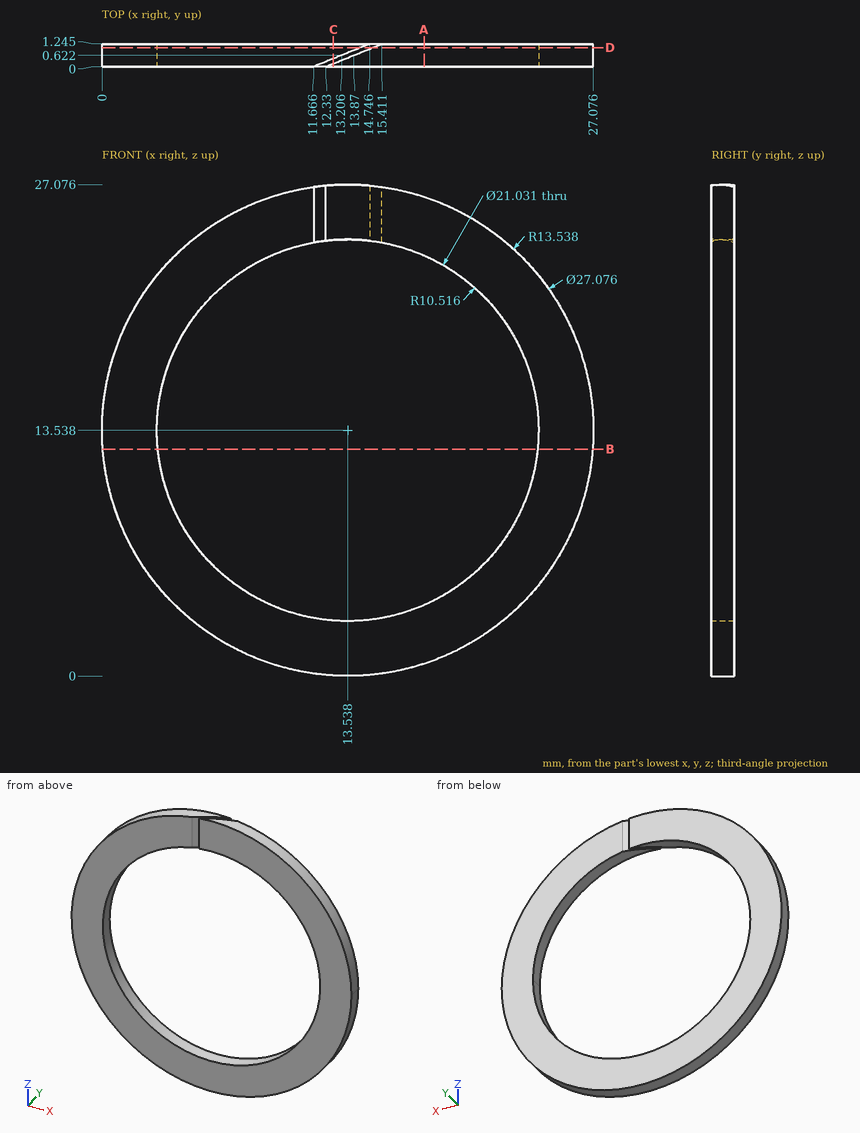
Answer from the drawing. Dimensions are ordinates in mm from the lowest x, y and z of the part. Coordinates: 2 decimals unless noted, no trailing zeros. Loops run counter-clockwise (first coordinate to the right, second up) from the corner with the lowest first, then second, coordinate; pieces in that order, holes last. Notation, with made-up numbers: (63.25, 7.5) -> (85.25, 7.5) arc R16 ccw to (85.25, 34.5) -> close; hole circle Ø1 at (44.25, -17.5). An arc over 180 degrees is marked (long way). Answer in a Markdown table with one row per item.
Item 1: This flat-tipped pin is pushed along its axis until it touches: P1, Ø12, axis at x = 17.5, z = 15.5, coming from the -Y side. Where does it stop, or does it pass through?
Returned:
| item | result |
|---|---|
| P1 | passes through |
Item 2: A cutting plane is placed at B-B on z = 12.5. Determine the outline of the cut face in (x, y) (1 decimal).
Returned:
| item | result |
|---|---|
| outline | (0, 0) -> (3.1, 0) -> (3.1, 1.2) -> (0, 1.2) -> close; (24, 0) -> (27, 0) -> (27, 1.2) -> (24, 1.2) -> close |
Item 3: Straight lines are drawn through the part: line 1 along Z through (x, y) = (13.5, 0.85); line 2 along Z through (x, y) = (17.25, 0.65); line 3 along X through (y, z) = (1, 19.5) (1 decimal). For each, find the intervals that lie inside material, in ascending order. Write a range as [from, to].
Returned:
| item | result |
|---|---|
| line 1 | z = [0, 3.02], [24.05, 27.08] |
| line 2 | z = [0.52, 3.7], [23.38, 26.56] |
| line 3 | x = [1.4, 4.9], [22.2, 25.7] |
Item 4: A cutting plane is placed at D-D on y = 1.05. Determine the outline of the cut face in (x, z) (1 decimal).
Returned:
| item | result |
|---|---|
| outline | (14.3, 24) -> (14.3, 27.1) arc R13.5 ccw (long way) to (14.9, 27) -> (14.9, 24) arc R10.5 cw (long way) to start |
Item 5: A cutting plane is placed at A-A on x = 17.75. Determine the outline of the cut face in (y, z) (1 decimal).
Returned:
| item | result |
|---|---|
| outline | (0, 0.7) -> (1.2, 0.7) -> (1.2, 3.9) -> (0, 3.9) -> close; (0, 23.2) -> (1.2, 23.2) -> (1.2, 26.4) -> (0, 26.4) -> close |
Item 6: A cutting plane is placed at C-C on x = 12.75. Give the number of separate pieces and of enclosed holes in the cut face.
Returned:
| item | result |
|---|---|
| separate pieces | 3 |
| enclosed holes | 0 |
